```python
from build123d import *

# Parameters (mm, degrees)
F0_W     = 2
F0_H     = 15
F1_DEPTH = 25
F2_W     = 53
F2_H     = 15
F3_DEPTH = 0.5


with BuildPart() as f1:
    # F0 (on Top) → F1 (new body)
    with BuildSketch(Plane.XY):
        with Locations((-47.719786, 0)):
            Rectangle(F0_W, F0_H)
        with Locations((-40.719786, 0)):
            Rectangle(F0_W, F0_H)
        with Locations((-23.719786, 0)):
            Rectangle(F0_W, F0_H)
        with Locations((3.280214, 0)):
            Rectangle(F0_W, F0_H)
    extrude(amount=F1_DEPTH)

    # F2 (on face) → F3 (join)
    with BuildSketch(Plane.XY.offset(25)):
        with Locations((-22.219786, 0)):
            Rectangle(F2_W, F2_H)
    extrude(amount=F3_DEPTH)


solid = f1.part
```
CAD build for the part. Positions are in the model's coordinates, mm. A direction names the side the tool comes from. Round coordinates to 2 decimals unless told otherwise and drop trailing zeros. Write each loop counter-clockwise with the first axis right and the second up, starting at its lowest first coordinate (ties: lowest second). Pieces come first, ordered by that corner, then holes. Notation, with made-up numbers: (-26, 60.5) -> (-18, 60.5) arc R26 cw to (-18, 84.5) -> close; hole circle Ø11 at (69, 72). An arc over 180 degrees is marked (long way). Answer in a Markdown table with one row per item. Add a question column.
Item 1: Saw through at B-B, the plane y = -6.25. Write the cut outline in (x, z), then the cut area to 4 significant figures.
Item 2: Drop a flat-ended pin along its axis: pin 1 Ø8 at (x, y) = (-12.5, -4.5) entering from -Z. Give the stop position or say it passes through.
Item 3: Drill centre lines: line 1 (X direction, y = -0.25, z = 22.5); line 2 (Z direction, x = -38, y = -0.25). Where is each one in solid material? Low to high. Write a range as from..to.
Item 4: Saw through at C-C, the plane x = -27. Write the cut outline in (y, z), then the cut area to 3 significant figures.
Item 5: Saw through at A-A, the plane z = 12.75. Write the cut outline in (x, y).
Item 6: Mould opens along X. For faces 1 (the face through (4.28, 0, 13)), 2 (the face through (-48.72, 0, 13)), 3 (the face through (-46.72, 0, 12)), 4 (the face through (3, 0, 0)) say: pulls with the +X half, pulls with the -X half, needs draft (parallel to the pull), parting line crosses it, or undercut.
Item 7: Which spindle directions (+Z, -Z, +X, -X, +Y, -Y) get a long thin tool onto all of the face, cutting with end or side? Do faces 5 (the face through (-48, 0, 0)), 6 (the face through (-24.72, 0, 12)). Say none if no direction does.
Findings below:
| question | item | result |
|---|---|---|
| 1 | outline | (-48.72, 0) -> (-46.72, 0) -> (-46.72, 25) -> (-41.72, 25) -> (-41.72, 0) -> (-39.72, 0) -> (-39.72, 25) -> (-24.72, 25) -> (-24.72, 0) -> (-22.72, 0) -> (-22.72, 25) -> (2.28, 25) -> (2.28, 0) -> (4.28, 0) -> (4.28, 25.5) -> (-48.72, 25.5) -> close |
| 1 | area | 226.5 mm^2 |
| 2 | pin 1 | stops at z = 25 |
| 3 | line 1 | x = -48.72..-46.72, -41.72..-39.72, -24.72..-22.72, 2.28..4.28 |
| 3 | line 2 | z = 25..25.5 |
| 4 | outline | (-7.5, 25) -> (7.5, 25) -> (7.5, 25.5) -> (-7.5, 25.5) -> close |
| 4 | area | 7.50 mm^2 |
| 5 | outline | (-48.72, -7.5) -> (-46.72, -7.5) -> (-46.72, 7.5) -> (-48.72, 7.5) -> close; (-41.72, -7.5) -> (-39.72, -7.5) -> (-39.72, 7.5) -> (-41.72, 7.5) -> close; (-24.72, -7.5) -> (-22.72, -7.5) -> (-22.72, 7.5) -> (-24.72, 7.5) -> close; (2.28, -7.5) -> (4.28, -7.5) -> (4.28, 7.5) -> (2.28, 7.5) -> close |
| 6 | face 1 | pulls with the +X half |
| 6 | face 2 | pulls with the -X half |
| 6 | face 3 | undercut |
| 6 | face 4 | needs draft |
| 7 | face 5 | -Z, +X, -X, +Y, -Y |
| 7 | face 6 | -Z, +Y, -Y |
